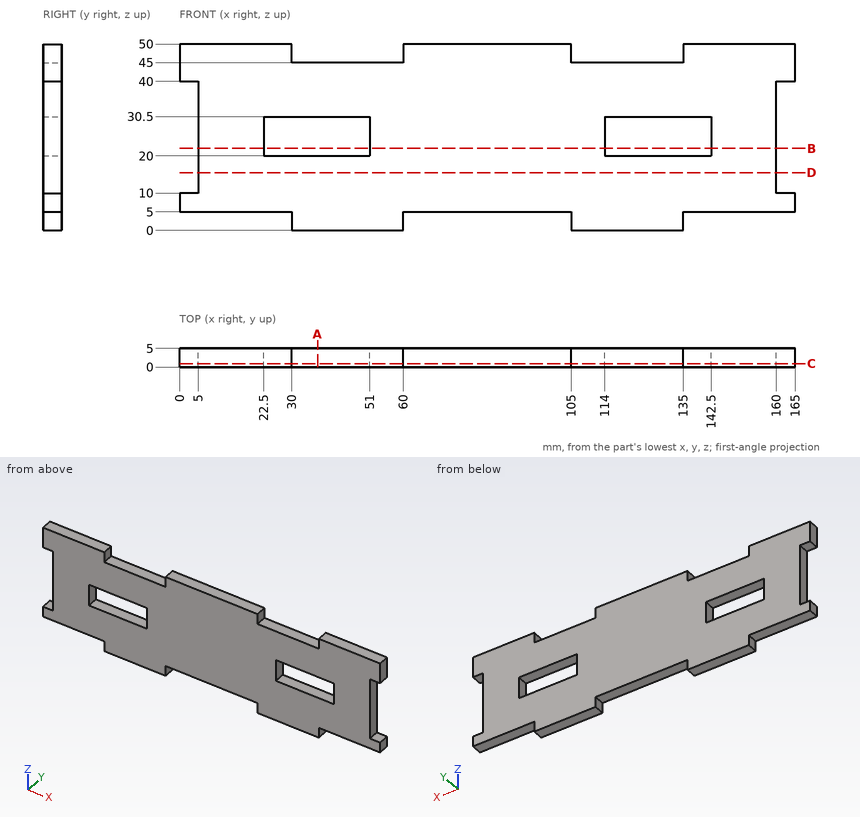
Study the drawing (mm; zero at the part's minimum x, y, z) and answer. Give positions to 0.01 mm unless a question says otherwise; leave off trailing zeros. Loops run counter-clockwise (first coordinate to the right, second up) from the corner with the lowest first, then second, coordinate; pieces in that order, holes last. Notation, with made-up numbers: (33.25, 5.5) -> (40.25, 5.5) arc R23 ccw to (40.25, 16.5) -> close; hole circle Ø2 at (3.25, 88.5). An arc over 180 degrees is marked (long way). Use a Markdown table: item, result. Add a question column.
1) The part is cut by section D-D, the plane z = 15.5. Determine the outline of the cut face in (x, y).
2) The part is cut by section B-B, the plane z = 22. Determine the outline of the cut face in (x, y).
3) Consider line 1 along X through (y, z) = (4.7, 24); line 2 along X through (y, z) = (0.5, 47); line 3 along Z through (x, y) = (44, 2.65). Determine where each line is inside the solid, lowest interval first.
4) The part is cut by section C-C, the plane y = 0.95. Count the separate pieces of the cut face and the enclosed holes in it, plus the area to 3 significant figures.
5) Each of these flat-tipped pins is pushed along its axis until it touches: P1, Ø1.5, axis at x = 91, y = 1.5, coming from the -Z side; P2, Ø2.5, axis at y = 3.5, z = 3, coming from the -X side; P3, Ø2.5, axis at y = 2, z = 26.5, coming from the -X side; P4, Ø2.5, axis at x = 42, y = 2.5, coming from the -Z side. Where does it stop, or does it pass through?
6) The part is cut by section A-A, the plane x = 37. Determine the outline of the cut face in (y, z), plus the area to 4 significant figures.
Reported:
| question | item | result |
|---|---|---|
| 1 | outline | (5, 0) -> (160, 0) -> (160, 5) -> (5, 5) -> close |
| 2 | outline | (5, 0) -> (22.5, 0) -> (22.5, 5) -> (5, 5) -> close; (51, 0) -> (114, 0) -> (114, 5) -> (51, 5) -> close; (142.5, 0) -> (160, 0) -> (160, 5) -> (142.5, 5) -> close |
| 3 | line 1 | x = 5 to 22.5, 51 to 114, 142.5 to 160 |
| 3 | line 2 | x = 0 to 30, 60 to 105, 135 to 165 |
| 3 | line 3 | z = 0 to 20, 30.5 to 45 |
| 4 | separate pieces | 1 |
| 4 | enclosed holes | 2 |
| 4 | area | 6,530 mm^2 |
| 5 | P1 | stops at z = 5 |
| 5 | P2 | stops at x = 30 |
| 5 | P3 | stops at x = 5 |
| 5 | P4 | stops at z = 0 |
| 6 | outline | (0, 0) -> (5, 0) -> (5, 20) -> (0, 20) -> close; (0, 30.5) -> (5, 30.5) -> (5, 45) -> (0, 45) -> close |
| 6 | area | 172.5 mm^2 |
